Part model, mm, in its own coordinate system. A direction names the side the tool comes from. Give positions to 0.01 mm unless a question says otherwise; leave off trailing zeros. Order: outer loops, then holes, each group sorted by start corner. A loop starts at its lowest first (then second) coordinate and runs counter-clockwise, first axis right, second up. Notation, with made-up numbers: (16.5, -39.5) - (57.5, -39.5) arc R35 ccw to (57.5, -3.5) - close; hole circle Ø7 at (-4, 17.5). An arc over 180 degrees is marked (long way). One line per item, written item: value.
```python
from build123d import *

# Parameters (mm, degrees)
BOSS_EXTRUDE1_DEPTH = 39.84
CUT_EXTRUDE1_REACH  = 62.108
SKETCH3_W           = 10
SKETCH3_H           = 2.74
BOSS_EXTRUDE2_DEPTH = 2.74


with BuildPart() as part:
    # Sketch1 → Boss-Extrude1 (new body)
    with BuildSketch(Plane(origin=(0, 0, 0), x_dir=(-1, 0, 0), z_dir=(0, 1, 0))):
        Polygon((-12.003904286, -2.835509232), (-12.003904286, -5.835509232), (27.996095714, -5.835509232), (27.996095714, -2.835509232), (-8.539802671, -2.835509232), (10.594171925, 30.305506919), (7.996095714, 31.805506919), align=None)
    extrude(amount=BOSS_EXTRUDE1_DEPTH)

    # Sketch2 → Cut-Extrude1 (cut, up to next)
    with BuildSketch(Plane(origin=(7.775116701, 0, 4.48896572), x_dir=(0, 1, 0), z_dir=(0.8660254037844364, 0, 0.5000000000000038)), mode=Mode.PRIVATE) as cut_extrude1_sk1:
        with BuildLine():
            Line((6, 21.542424829), (6, 11.542424829))
            ThreePointArc((6, 11.542424829), (8.64, 8.902424829), (11.28, 11.542424829))
            Line((11.28, 11.542424829), (11.28, 21.542424829))
            Line((11.28, 21.542424829), (12.45, 22.712424829))
            Line((12.45, 22.712424829), (12.45, 31.542424829))
            Line((12.45, 31.542424829), (11.28, 31.542424829))
            Line((11.28, 31.542424829), (6, 31.542424829))
            Line((6, 31.542424829), (4.83, 31.542424829))
            Line((4.83, 31.542424829), (4.83, 22.712424829))
            Line((4.83, 22.712424829), (6, 21.542424829))
        make_face()
    cut_extrude1_tool1 = extrude(cut_extrude1_sk1.sketch, amount=-CUT_EXTRUDE1_REACH, mode=Mode.PRIVATE) & part.part
    # Sketch2 → Cut-Extrude1 (cut, up to next)
    with BuildSketch(Plane(origin=(7.775116701, 0, 4.48896572), x_dir=(0, 1, 0), z_dir=(0.8660254037844364, 0, 0.5000000000000038)), mode=Mode.PRIVATE) as cut_extrude1_sk2:
        with BuildLine():
            Line((22.56, 21.542424829), (22.56, 11.542424829))
            ThreePointArc((22.56, 11.542424829), (19.92, 8.902424829), (17.28, 11.542424829))
            Line((17.28, 11.542424829), (17.28, 21.542424829))
            Line((17.28, 21.542424829), (16.11, 22.712424829))
            Line((16.11, 22.712424829), (16.11, 31.542424829))
            Line((16.11, 31.542424829), (17.28, 31.542424829))
            Line((17.28, 31.542424829), (22.56, 31.542424829))
            Line((22.56, 31.542424829), (23.73, 31.542424829))
            Line((23.73, 31.542424829), (23.73, 22.712424829))
            Line((23.73, 22.712424829), (22.56, 21.542424829))
        make_face()
    cut_extrude1_tool2 = extrude(cut_extrude1_sk2.sketch, amount=-CUT_EXTRUDE1_REACH, mode=Mode.PRIVATE) & part.part
    # Sketch2 → Cut-Extrude1 (cut, up to next)
    with BuildSketch(Plane(origin=(7.775116701, 0, 4.48896572), x_dir=(0, 1, 0), z_dir=(0.8660254037844364, 0, 0.5000000000000038)), mode=Mode.PRIVATE) as cut_extrude1_sk3:
        with BuildLine():
            Line((33.84, 21.542424829), (33.84, 11.542424829))
            ThreePointArc((33.84, 11.542424829), (31.2, 8.902424829), (28.56, 11.542424829))
            Line((28.56, 11.542424829), (28.56, 21.542424829))
            Line((28.56, 21.542424829), (27.39, 22.712424829))
            Line((27.39, 22.712424829), (27.39, 31.542424829))
            Line((27.39, 31.542424829), (28.56, 31.542424829))
            Line((28.56, 31.542424829), (33.84, 31.542424829))
            Line((33.84, 31.542424829), (35.01, 31.542424829))
            Line((35.01, 31.542424829), (35.01, 22.712424829))
            Line((35.01, 22.712424829), (33.84, 21.542424829))
        make_face()
    cut_extrude1_tool3 = extrude(cut_extrude1_sk3.sketch, amount=-CUT_EXTRUDE1_REACH, mode=Mode.PRIVATE) & part.part
    add(cut_extrude1_tool1.solids().sort_by_distance((-2.97705, 8.64, 23.112265))[0], mode=Mode.SUBTRACT)
    add(cut_extrude1_tool2.solids().sort_by_distance((-2.97705, 19.92, 23.112265))[0], mode=Mode.SUBTRACT)
    add(cut_extrude1_tool3.solids().sort_by_distance((-2.97705, 31.2, 23.112265))[0], mode=Mode.SUBTRACT)

    # Sketch3 → Boss-Extrude2 (add)
    with BuildSketch(Plane(origin=(0, 0, -5.835509232), x_dir=(1, 0, 0), z_dir=(0, 0, -1))):
        with Locations((-7.996095714, -1.37)):
            Rectangle(SKETCH3_W, SKETCH3_H)
        with Locations((-7.996095714, -38.47)):
            Rectangle(SKETCH3_W, SKETCH3_H)
    extrude(amount=BOSS_EXTRUDE2_DEPTH)


solid = part.part
```
1) Slice it at C-C on z = 17.5. Write the cut outline in (x, y).
Answer:
outline: (-3.2, 0) - (0.26, 0) - (0.26, 6) - (-3.2, 6) - close; (-3.2, 11.28) - (0.26, 11.28) - (0.26, 17.28) - (-3.2, 17.28) - close; (-3.2, 22.56) - (0.26, 22.56) - (0.26, 28.56) - (-3.2, 28.56) - close; (-3.2, 33.84) - (0.26, 33.84) - (0.26, 39.84) - (-3.2, 39.84) - close
2) Wall check: line 1 along Z through (x, y) = (0.5, 31); line 2 along Z through (x, y) = (8, 8); line 3 along Z through (x, y) = (5, 17.5). Give the ranges that are in metal, low to high. Write a range as [from, to].
Answer:
line 1: z = [-5.84, -2.84]
line 2: z = [-5.84, -2.84], [-1.9, 4.1]
line 3: z = [-5.84, -2.84], [3.3, 9.3]
3) Which spindle directions (+Z, -Z, +X, -X, +Y, -Y) get a long thin tool onto all of the face, cutting with end or side? Do faces 1 (the face through (-8, 1, -8.576)), 2 (the face through (-12.996, 1, -7)), 3 (the face through (-4.565, 11.857, 22.905)). Say none if no direction does.
Answer:
face 1: -Z, +X, -X, +Y, -Y
face 2: -Z, -X, +Y, -Y
face 3: +Z, -X
4) Two-plate mould, pull along Y, no slides. Class faces 4 (the face through (-2.996, 38, -7)), 5 (the face through (-3, 39.84, -3)), 6 (the face through (-2, 22.56, 18)): pulls with the +Y half, pulls with the -Y half, needs draft (parallel to the pull), parting line crosses it, or undercut.
Answer:
face 4: needs draft
face 5: pulls with the +Y half
face 6: undercut
5) Slice it at A-A on y = 36.5. Write the cut outline in (x, z), then the cut area to 3 significant figures.
Answer:
outline: (-28, -5.84) - (12, -5.84) - (12, -2.84) - (-8, 31.81) - (-10.59, 30.31) - (8.54, -2.84) - (-28, -2.84) - close
area: 237 mm2
6) Drop flat-ended pins along their axis: P1, Ø6, axis at x = 3.5, y = 24.5, coming from the +Z side; P2, Ø1.4, axis at y = 38, z = -7, coming from the +X side; P3, Ø6, axis at y = 28.5, z = 6.5, coming from the -X side; P4, Ø2, axis at y = 32.5, z = 16, coming from the -X side. Give the stop position or say it passes through.
Answer:
P1: stops at z = 17.09
P2: stops at x = -3
P3: stops at x = 1.42
P4: passes through
7) Slice it at D-D on y = 7. Write the cut outline in (x, z), then the cut area to 3 significant figures.
Answer:
outline: (-28, -5.84) - (12, -5.84) - (12, -2.84) - (3.04, 12.69) - (0.44, 11.19) - (8.54, -2.84) - (-28, -2.84) - close
area: 171 mm2
8) Slice it at B-B on x = -9.5. Write the cut outline in (y, z).
Answer:
outline: (0, -8.58) - (2.74, -8.58) - (2.74, -5.84) - (37.1, -5.84) - (37.1, -8.58) - (39.84, -8.58) - (39.84, -2.84) - (0, -2.84) - close; (0, 28.41) - (4.83, 28.41) - (4.83, 30.94) - (0, 30.94) - close; (12.45, 28.41) - (16.11, 28.41) - (16.11, 30.94) - (12.45, 30.94) - close; (23.73, 28.41) - (27.39, 28.41) - (27.39, 30.94) - (23.73, 30.94) - close; (35.01, 28.41) - (39.84, 28.41) - (39.84, 30.94) - (35.01, 30.94) - close
